Geometry check sheet. Reference: the model listing, model coordinates, mm. A direction names the side the tool comes from. Give positions to 0.01 mm unless a question says otherwise; leave off trailing zeros. Order: outer loops, then holes, each group sorted by start corner. A loop starts at its lowest first (then second) coordinate and runs counter-clockwise, first axis right, second up. Notation, with made-up numbers: M -15.75,20 L 12.25,20 A22 ccw 12.25,47 Z; hole C 67,86 d11. An arc over 180 degrees is marked long. Put each result on its own line as item: value. Start each with the question number.
Q1. Section check B-B on y = 20. Record the cut outline in (x, z).
Q2. Access from +Z, -Z, +X, -X, +Y, -Y to the whole of each face (thin tool, end or side, straight path). Record for faces 1 (the cylindrical face through (79.1, 16, 4.9)), 2 (the flat face through (0, 52, -5)).
Q3. Section check A-A on z = -3.75. Record the cut outline in (x, y).
Q4. Go/stop test with flat-tipped pins: pin 1 (5 mm diameter, centred on y = 41, z = 1, fed in from +X); pin 2 (1 mm diameter, centred on x = 126.5, y = 71.5, fed in from +Z). Record where each tip stops, or that it passes through.
Q5. Section check C-C on x = 43. Record the cut outline in (y, z), then the cut area to 3 significant figures.
Q6. Mould release check, pull along X, two halves, no side actions. Record for faces 3 (the flat face through (10, 52, -3)), 4 (the flat face through (140, 52, -5)), 5 (the flat face through (77, 12, 10)): +X half, -X half, draft (parallel to the pull), parting line (faces both ways), or undercut.
Q7. Material ranges on L1, parallel to X at y = 71.5, z = 7.25; L2, parallel to Y at x = 58.5, z = -1; L3, parallel to X at y = 22, z = -1, recorded low to high.
```python
from build123d import *

# Parameters (mm, degrees)
F0_W     = 140
F0_H     = 105
F1_DEPTH = 10
F2_R     = 3
F2_R_2   = 1
F3_DEPTH = 10
F4_W     = 56
F4_H     = 85
F5_DEPTH = 6


with BuildPart() as f1:
    # F0 (on Top) → F1 (new body)
    with BuildSketch(Plane.XY):
        with Locations((70, 52.5)):
            Rectangle(F0_W, F0_H)
    extrude(amount=-F1_DEPTH)

    # F2 (on Top) → F3 (join)
    with BuildSketch(Plane.XY):
        with Locations((77.444687, 71.503997)):
            Circle(F2_R)
        with Locations((77.444687, 71.503997)):
            Circle(F2_R_2, mode=Mode.SUBTRACT)
        with Locations((126.459315, 71.503997)):
            Circle(F2_R)
        with Locations((126.459315, 71.503997)):
            Circle(F2_R_2, mode=Mode.SUBTRACT)
        with Locations((126.459315, 13.496778)):
            Circle(F2_R)
        with Locations((126.459315, 13.496778)):
            Circle(F2_R_2, mode=Mode.SUBTRACT)
        with Locations((77.444687, 13.496778)):
            Circle(F2_R)
        with Locations((77.444687, 13.496778)):
            Circle(F2_R_2, mode=Mode.SUBTRACT)
    extrude(amount=F3_DEPTH)

    # F4 (on face) → F5 (cut)
    with BuildSketch(Plane.XY):
        with Locations((38, 52.5)):
            Rectangle(F4_W, F4_H)
    extrude(amount=-F5_DEPTH, mode=Mode.SUBTRACT)


solid = f1.part
```
Results found:
1. outline: M 0,-10 L 140,-10 L 140,0 L 66,0 L 66,-6 L 10,-6 L 10,0 L 0,0 Z
2. face 1: +Z
2. face 2: +Z, -Z, -X, +Y, -Y
3. outline: M 0,0 L 140,0 L 140,105 L 0,105 Z; hole M 10,10 L 66,10 L 66,95 L 10,95 Z
4. pin 1: stops at x = 140
4. pin 2: stops at z = 0
5. outline: M 0,-10 L 105,-10 L 105,0 L 95,0 L 95,-6 L 10,-6 L 10,0 L 0,0 Z
5. area: 540 mm^2
6. face 3: undercut
6. face 4: +X half
6. face 5: draft
7. L1: x = 74.44 to 76.44, 78.44 to 80.44, 123.46 to 125.46, 127.46 to 129.46
7. L2: y = 0 to 10, 95 to 105
7. L3: x = 0 to 10, 66 to 140
